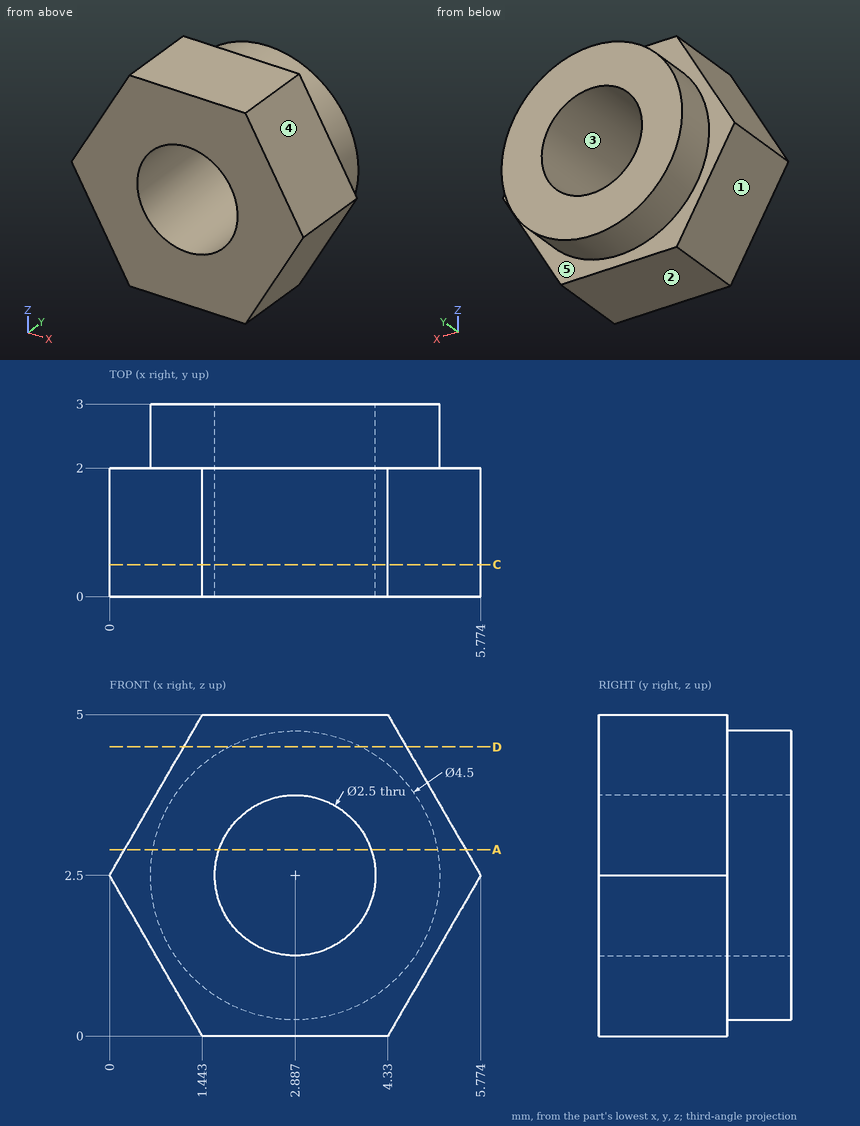
Geometry check sheet. Reference: drawing and pictorial views, mm from the part's lowest x, y, z. A direction names the side the tool comes from. Round coordinates to 2 decimals unless told otherwise and drop trailing zeros. Order: outer loops, then holes, each group sorted by start corner. A loop starts at its lowest first (then second) coordinate and runs counter-clockwise, first axis right, second up. Notation, with made-up numbers: (2, 33) - (21, 33) arc R25 ccw to (21, 46) - close; hole circle Ø3 at (68, -19). An arc over 180 degrees is marked (long way). Use a Markdown table: item, result. Add a question column.
1) Mould release check, pull along X, two halves, no side actions. Record for the marked faces 1, 2 and 3: released by +X, released by -X, zero draft, split by the parting line, or undercut.
2) Section check C-C (y = 0.5). Record the cut outline in (x, z).
3) Set-up check for the marked faces 4 and 5: record each of +Z, -Z, +X, -X, +Y, -Y from which the full face is reachable in a straight line by a thin tool's end or side.
4) Thickness scan on line 1 along Z through (x, y) = (2.4, 1.5); line 2 along X through (y, z) = (0.45, 2.8) (1 decimal); line 3 along X through (y, z) = (1.7, 1.5) (1 decimal). Record the ranges inside material, lowest first.
5) Section check D-D (z = 4.5). Record the cut outline in (x, y) (1 decimal).
6) Section check A-A (z = 2.9). Record the cut outline in (x, y).
Established:
| question | item | result |
|---|---|---|
| 1 | face 1 | released by -X |
| 1 | face 2 | zero draft |
| 1 | face 3 | undercut |
| 2 | outline | (0, 2.5) - (1.44, 0) - (4.33, 0) - (5.77, 2.5) - (4.33, 5) - (1.44, 5) - close; hole circle Ø2.5 at (2.89, 2.5) |
| 3 | face 4 | +Z, +X, +Y, -Y |
| 3 | face 5 | +Y |
| 4 | line 1 | 0 to 1.35, 3.65 to 5 |
| 4 | line 2 | 0.2 to 1.7, 4.1 to 5.6 |
| 4 | line 3 | 0.6 to 2.1, 3.6 to 5.2 |
| 5 | outline | (1.2, 0) - (4.6, 0) - (4.6, 2) - (3.9, 2) - (3.9, 3) - (1.9, 3) - (1.9, 2) - (1.2, 2) - close |
| 6 | outline | (0.23, 0) - (1.7, 0) - (1.7, 3) - (0.67, 3) - (0.67, 2) - (0.23, 2) - close; (4.07, 0) - (5.54, 0) - (5.54, 2) - (5.1, 2) - (5.1, 3) - (4.07, 3) - close |
